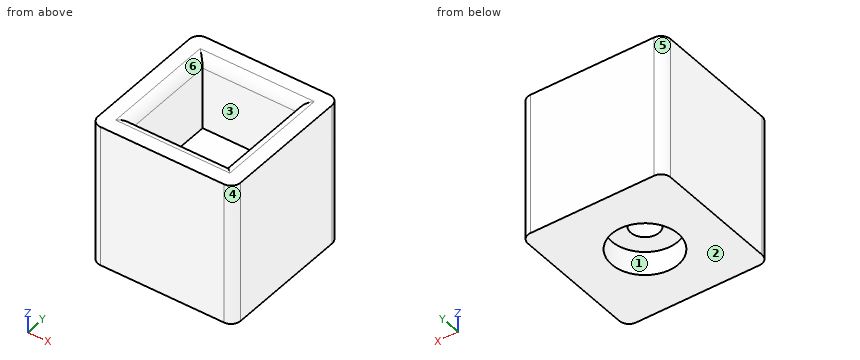
```python
from build123d import *

# Parameters (mm, degrees)
F0_W     = 30
F0_H     = 30
F1_DEPTH = 30
F2_W     = 20
F2_H     = 20
F3_DEPTH = 15
F4_R     = 3
F5_DEPTH = 25
F6_R     = 7
F7_DEPTH = 5
F8_R     = 2


with BuildPart() as f1:
    # F0 (on Top) → F1 (new body)
    with BuildSketch(Plane.XY):
        with Locations((15, 15)):
            Rectangle(F0_W, F0_H)
    extrude(amount=F1_DEPTH)

    # F2 (on face) → F3 (cut)
    with BuildSketch(Plane.XY.offset(30)):
        with Locations((15, 15)):
            Rectangle(F2_W, F2_H)
    extrude(amount=-F3_DEPTH, mode=Mode.SUBTRACT)

    # F4 (on face) → F5 (cut)
    with BuildSketch(Plane(origin=(0, 0, 0), x_dir=(1, 0, 0), z_dir=(0, 0, -1))):
        with Locations((15, -15)):
            Circle(F4_R)
    extrude(amount=-F5_DEPTH, mode=Mode.SUBTRACT)

    # F6 (on face) → F7 (cut)
    with BuildSketch(Plane(origin=(0, 0, 0), x_dir=(1, 0, 0), z_dir=(0, 0, -1))):
        with Locations((15, -15)):
            Circle(F6_R)
    extrude(amount=-F7_DEPTH, mode=Mode.SUBTRACT)

    # F8
    f8_edges = [f1.edges().sort_by_distance(p)[0] for p in [
        (5, 15, 30),
        (15, 25, 30),
        (25, 15, 30),
        (15, 5, 30),
        (30, 0, 15),
        (30, 30, 15),
        (0, 0, 15),
        (0, 30, 15),
    ]]
    fillet(f8_edges, radius=F8_R)


solid = f1.part
```
Geometry: final body of the model. Coordinates: model frame, mm. Face numbers are marked on the shaded views. A direction names the side the tool comes from. Give positions to 0.01 mm unless a question says otherwise; leave off trailing zeros. Loops run counter-clockwise (first coordinate to the right, second up) from the corner with the lowest first, then second, coordinate; pieces in that order, holes last. Notation, with made-up numbers: (-13, 19.25) -> (17, 19.25) arc R19 ccw to (17, 28.25) -> close; hole circle Ø8 at (-10.5, -2.5). An arc over 180 degrees is marked (long way). Return JSON: item names as keys, results as strings.
Item 1: Pin query (flat end, axial travel): P1, Ø5.5, axis at x = 15, y = 15, coming from the -Z side; P2, Ø12.5, axis at x = 15, y = 15, coming from the +Z side. Return the tip coordinate at first contact, or that it passes through.
Filled in:
{"P1": "through", "P2": "z = 15"}
Item 2: Section D-D, the plane x = 21.25. Output: boundary loops of the cut face in (y, z), plus the area to 3 significant figures.
Filled in:
{"outline": "(0, 0) -> (11.85, 0) -> (11.85, 5) -> (18.15, 5) -> (18.15, 0) -> (30, 0) -> (30, 30) -> (27, 30) arc R2 ccw to (25, 28) -> (25, 15) -> (5, 15) -> (5, 28) arc R2 ccw to (3, 30) -> (0, 30) -> close", "area": "567 mm^2"}
Item 3: Line query: line 1 (Y direction, x = 24.25, z = 24); line 2 (Y direction, x = 15, z = 1.05). Output: solid intervals per line, ascending.
Filled in:
{"line 1": "0 to 5, 25 to 30", "line 2": "0 to 8, 22 to 30"}
Item 4: Section B-B, the plane z = 16.25. Output: boundary loops of the cut face in (x, y), plus the area to 3 significant figures.
Filled in:
{"outline": "(0, 2) arc R2 ccw to (2, 0) -> (28, 0) arc R2 ccw to (30, 2) -> (30, 28) arc R2 ccw to (28, 30) -> (2, 30) arc R2 ccw to (0, 28) -> close; hole (5, 5) -> (25, 5) -> (25, 25) -> (5, 25) -> close", "area": "497 mm^2"}
Item 5: Access query for the marked faces 1, 2 and 3. Directions: +Z, -Z, +X, -X, +Y, -Y. A direction counts if a zero-diameter tool reaches every point of the face in a straight line with its end or side. Return the directions, or none.
Filled in:
{"face 1": "-Z", "face 2": "-Z, +X, -X, +Y, -Y", "face 3": "+Z"}
Item 6: Section A-A, the plane x = 15. Output: boundary loops of the cut face in (y, z).
Filled in:
{"outline": "(0, 0) -> (8, 0) -> (8, 5) -> (12, 5) -> (12, 15) -> (5, 15) -> (5, 28) arc R2 ccw to (3, 30) -> (0, 30) -> close; (18, 5) -> (22, 5) -> (22, 0) -> (30, 0) -> (30, 30) -> (27, 30) arc R2 ccw to (25, 28) -> (25, 15) -> (18, 15) -> close"}
Item 7: Mould query, pull axis X, two halves, no side actions, for the marked faces 4, 5 and 6. Classes: released by +X, released by -X, zero draft, split by the parting line, or undercut.
Filled in:
{"face 4": "released by +X", "face 5": "released by -X", "face 6": "undercut"}
